Part model, mm, in its own coordinate system. A direction names the side the tool comes from. Round coordinates to 2 decimals unless told otherwise and drop trailing zeros. Write each loop counter-clockwise with the first axis right and the second up, starting at its lowest first coordinate (ties: lowest second). Pieces come first, ordered by that corner, then holes. Notation, with made-up numbers: M -11.75,-22.5 L 47.25,-22.5 A27 ccw 47.25,0.5 Z; hole C 0.25,54 d5. An arc over 180 degrees is marked long. One line per question, with ' | ' between items. Start each with the question number.
1) Wall check: probe 1 along Z at (x, y) = (68, 7); probe 2 along X at (y, z) = (18, -121.5); probe 3 along Z at (x, y) = (68.35, 7.5). Give the ranges that are in metal, low to high. Write a range as [from, to].
2) Drop flat-ended pins along their axis: pin 1 Ø1.5 at (x, z) = (77.5, -23) entering from +Y; pin 2 Ø1 at (x, y) = (96.5, 8.5) entering from -Z; pin 3 Ø4.5 at (x, y) = (45.5, 8) entering from -Z; pin 4 Ø3 at (y, z) = (7.5, -31.25) entering from -X. Give the stop position or say it passes through.
3) Mould opens along Z. For faces 1 (the face through (113, 10, -98.995)), 2 (the face through (69, 7, -138)), 3 (the face through (58, 2, -170)), 4 (the face through (75.29, 7, -100)) say: pulls with the +Z half, pulls with the -Z half, needs draft (parallel to the pull), parting line crosses it, or undercut.
4) Saw through at C-C (z = -122.5). List the corners of the cut face in (x, y).
5) Saw through at B-B (y = 26.5). List the corners of the cut face in (x, z), plus the area to 3 significant figures.
6) Tool access for faces 5 (the face through (45, 7, -48)), 6 (the face through (69.5, 6, -156)), 7 (the face through (112.782, 26.678, -66.163)), 8 (the face through (43.5, 7, -151)), 9 (the face through (96, 7, -102.576)): list every direction of +Z, -Z, +X, -X, +Y, -Y with a clear straight run to the whole face (end or side of a thin tool).
```python
from build123d import *

# Parameters (mm, degrees)
SKETCH1_W                  = 110.5
SKETCH1_H                  = 170
SKETCH1_W_2                = 4.5
BOSS_EXTRUDE1_DEPTH        = 4
SKETCH1_4_W                = 4.5
SKETCH1_4_H                = 170
BOSS_EXTRUDE2_DEPTH        = 50
CUT_EXTRUDE1_DEPTH         = 4.5
SALIENTE_EXTRUIR1_DEPTH    = 7
SALIENTE_EXTRUIR2_DEPTH    = 7
CORTAR_EXTRUIR1_DEPTH      = 31
CORTAR_EXTRUIR1_DEPTH_BACK = 7
CORTAR_EXTRUIR2_DEPTH      = 2
CHAFL_N1_SIZE              = 4
CHAFL_N2_SIZE              = 4
CROQUIS5_R                 = 2.5
CORTAR_EXTRUIR3_DEPTH      = 23.7
CHAFL_N3_SIZE              = 4
SALIENTE_EXTRUIR4_DEPTH    = 7
CROQUIS8_W                 = 12
CROQUIS8_H                 = 8
CORTAR_EXTRUIR4_DEPTH      = 7
REDONDEO1_R                = 2


with BuildPart() as part:
    # Sketch1 → Boss-Extrude1 (new body)
    with BuildSketch(Plane(origin=(0, 0, 0), x_dir=(1, 0, 0), z_dir=(0, 1, 0))):
        with Locations((59.75, 85)):
            Rectangle(SKETCH1_W, SKETCH1_H)
        with Locations((2.25, 85)):
            Rectangle(SKETCH1_W_2, SKETCH1_H)
    extrude(amount=BOSS_EXTRUDE1_DEPTH)

    # Sketch1<4> → Boss-Extrude2 (add)
    with BuildSketch(Plane(origin=(0, 0, 0), x_dir=(1, 0, 0), z_dir=(0, 1, 0))):
        with Locations((2.25, 85)):
            Rectangle(SKETCH1_4_W, SKETCH1_4_H)
    boss_extrude2 = extrude(amount=BOSS_EXTRUDE2_DEPTH)

    # Sketch2 → Cut-Extrude1 (cut)
    with BuildSketch(Plane.ZY):
        Polygon((-134.204014838, 50), (-170, 4), (-182.392562203, 4), (-182.392562203, 57.402643918), (5.745866014, 57.402643918), (5.745866014, 4), (0, 4), align=None)
    cut_extrude1 = extrude(amount=-CUT_EXTRUDE1_DEPTH, mode=Mode.SUBTRACT)

    # Mirror1: Boss-Extrude2, Cut-Extrude1 across plane
    add(boss_extrude2.mirror(Plane(origin=(57.5, 0, 0), x_dir=(0, 0, 1), z_dir=(1, 0, 0))))
    add(cut_extrude1.mirror(Plane(origin=(57.5, 0, 0), x_dir=(0, 0, 1), z_dir=(1, 0, 0))), mode=Mode.SUBTRACT)

    # Sketch3 → Saliente-Extruir1 (add)
    with BuildSketch(Plane(origin=(0, 4, 0), x_dir=(1, 0, 0), z_dir=(0, 1, 0))):
        Polygon((57.5, 160), (47.5, 160), (47.5, 142), (47.5, 138), (43.5, 138), (43.5, 164), (57.5, 164), align=None)
    saliente_extruir1 = extrude(amount=SALIENTE_EXTRUIR1_DEPTH)

    # Croquis1 → Saliente-Extruir2 (add)
    with BuildSketch(Plane(origin=(0, 4, 0), x_dir=(1, 0, 0), z_dir=(0, 1, 0))):
        Polygon((57.5, 26), (57.5, 22), (43.5, 22), (43.5, 48), (47.5, 48), (47.5, 26), align=None)
    saliente_extruir2 = extrude(amount=SALIENTE_EXTRUIR2_DEPTH)

    # Simetría1: Saliente-Extruir1, Saliente-Extruir2 across plane
    add(saliente_extruir1.mirror(Plane(origin=(57.5, 11, -164), x_dir=(0, 0, 1), z_dir=(-1, 0, 0))))
    add(saliente_extruir2.mirror(Plane(origin=(57.5, 11, -164), x_dir=(0, 0, 1), z_dir=(-1, 0, 0))))

    # Croquis2 → Cortar-Extruir1 (cut, two sides: drawn at the far end of the back side and taken through both)
    with BuildSketch(Plane(origin=(47.5, 0, 0), x_dir=(0, 0, -1), z_dir=(1, 0, 0)).offset(-CORTAR_EXTRUIR1_DEPTH_BACK)):
        with BuildLine():
            Line((31.25, 9.974873734), (32.487436867, 8.737436867))
            ThreePointArc((32.487436867, 8.737436867), (31.25, 5.75), (30.012563133, 8.737436867))
            Line((30.012563133, 8.737436867), (31.25, 9.974873734))
        make_face()
        with BuildLine():
            Line((154.75, 9.974873734), (155.987436867, 8.737436867))
            ThreePointArc((155.987436867, 8.737436867), (154.75, 5.75), (153.512563133, 8.737436867))
            Line((153.512563133, 8.737436867), (154.75, 9.974873734))
        make_face()
    extrude(amount=CORTAR_EXTRUIR1_DEPTH + CORTAR_EXTRUIR1_DEPTH_BACK, mode=Mode.SUBTRACT)

    # Croquis4 → Cortar-Extruir2 (cut)
    with BuildSketch(Plane(origin=(71.5, 0, 0), x_dir=(0, 0, -1), z_dir=(1, 0, 0))):
        Polygon((158.069764048, 7.5), (156.409882024, 10.375), (153.090117976, 10.375), (151.430235952, 7.5), (153.090117976, 4.625), (156.409882024, 4.625), align=None)
        Polygon((29.590117976, 4.625), (27.930235952, 7.5), (29.590117976, 10.375), (32.909882024, 10.375), (34.569764048, 7.5), (32.909882024, 4.625), align=None)
    extrude(amount=-CORTAR_EXTRUIR2_DEPTH, mode=Mode.SUBTRACT)

    # Chaflán1
    chafl_n1_edges = [part.edges().sort_by_distance(p)[0] for p in [
        (57.5, 11, -26),
    ]]
    chamfer(chafl_n1_edges, length=CHAFL_N1_SIZE - 0.0001)  # a hair under: the kernel refuses the full size

    # Chaflán2
    chafl_n2_edges = [part.edges().sort_by_distance(p)[0] for p in [
        (57.5, 11, -160),
    ]]
    chamfer(chafl_n2_edges, length=CHAFL_N2_SIZE - 0.0001)  # a hair under: the kernel refuses the full size

    # Croquis5 → Cortar-Extruir3 (cut)
    with BuildSketch(Plane(origin=(0, 4, 0), x_dir=(1, 0, 0), z_dir=(0, 1, 0))):
        with Locations(Location((33.545716199, 107.830838948, 0), (0, 0, 270))):
            Circle(CROQUIS5_R)
        with Locations(Location((57.5, 51.866184435, 0), (0, 0, 270))):
            Circle(CROQUIS5_R)
        with Locations(Location((81.454283801, 107.830838948, 0), (0, 0, 270))):
            Circle(CROQUIS5_R)
    extrude(amount=-CORTAR_EXTRUIR3_DEPTH, mode=Mode.SUBTRACT)

    # Chaflán3
    chafl_n3_edges = [part.edges().sort_by_distance(p)[0] for p in [
        (57.5, 0, 0),
    ]]
    chamfer(chafl_n3_edges, length=CHAFL_N3_SIZE - 0.0001)  # a hair under: the kernel refuses the full size

    # Saliente-Extruir3: read off the stored shape, not the designer's step
    # Saliente-Extruir3: loft between two sections, ruled curve by curve
    saliente_extruir3_from = [
        Edge.make_line((89.622165017, 4, -44.992823986), (87.622165017, 4, -44.990685532)),
        Edge.make_line((89.66503142, 4, -53.010916957), (89.622165017, 4, -44.992823986)),
        Edge.make_line((89.66503142, 4, -53.010916957), (97.363741989, 4, -53.010916957)),
        Edge.make_line((97.363741989, 4, -53.010916957), (97.363741989, 4, -44.990685532)),
        Edge.make_line((97.363741989, 4, -44.990685532), (99.363741989, 4, -44.990685532)),
        Edge.make_line((99.363741989, 4, -44.990685532), (99.363741989, 4, -55.010916957)),
        Edge.make_line((99.363741989, 4, -55.010916957), (87.622165017, 4, -55.010916957)),
        Edge.make_line((87.622165017, 4, -44.990685532), (87.622165017, 4, -55.010916957)),
    ]
    saliente_extruir3_to = [
        Edge.make_line((89.622165017, 8.969440836, -41.812469009), (87.622165017, 8.969440836, -41.810330556)),
        Edge.make_line((89.66503142, 8.969440836, -49.83056198), (89.622165017, 8.969440836, -41.812469009)),
        Edge.make_line((89.66503142, 8.969440836, -49.83056198), (97.363741989, 8.969440836, -49.83056198)),
        Edge.make_line((97.363741989, 8.969440836, -49.83056198), (97.363741989, 8.969440836, -41.810330556)),
        Edge.make_line((97.363741989, 8.969440836, -41.810330556), (99.363741989, 8.969440836, -41.810330556)),
        Edge.make_line((99.363741989, 8.969440836, -41.810330556), (99.363741989, 8.969440836, -51.83056198)),
        Edge.make_line((99.363741989, 8.969440836, -51.83056198), (87.622165017, 8.969440836, -51.83056198)),
        Edge.make_line((87.622165017, 8.969440836, -41.810330556), (87.622165017, 8.969440836, -51.83056198)),
    ]
    saliente_extruir3 = Solid(Shell([*[Face.make_surface_from_curves(saliente_extruir3_from[k], saliente_extruir3_to[k]) for k in range(8)], Face(Wire(saliente_extruir3_from)), Face(Wire(saliente_extruir3_to))]))
    add(saliente_extruir3)

    # Croquis7 → Saliente-Extruir4 (add)
    with BuildSketch(Plane(origin=(0, 4, 0), x_dir=(1, 0, 0), z_dir=(0, 1, 0))):
        with BuildLine():
            Line((93.557674933, 100.575775557), (95.79024416, 100.575775557))
            Line((95.79024416, 100.575775557), (97.79024416, 100.575775557))
            Line((97.79024416, 100.575775557), (97.79024416, 102.575775557))
            Line((97.79024416, 102.575775557), (94.59024416, 102.575775557))
            ThreePointArc((94.59024416, 102.575775557), (92.49024416, 103.475775557), (90.39024416, 102.575775557))
            Line((90.39024416, 102.575775557), (75.29024416, 102.575775557))
            Line((75.29024416, 102.575775557), (75.29024416, 97.575775557))
            Line((75.29024416, 97.575775557), (77.29024416, 97.575775557))
            Line((77.29024416, 97.575775557), (77.29024416, 100.575775557))
            Line((77.29024416, 100.575775557), (80.20924649, 100.575775557))
            Line((80.20924649, 100.575775557), (91.59024416, 100.575775557))
            ThreePointArc((91.59024416, 100.575775557), (92.49024416, 99.675775557), (93.39024416, 100.575775557))
            Line((93.39024416, 100.575775557), (93.557674933, 100.575775557))
        make_face()
        with BuildLine():
            Line((94.726312137, 74.375775557), (97.79024416, 74.375775557))
            Line((97.79024416, 74.375775557), (97.79024416, 76.375775557))
            Line((97.79024416, 76.375775557), (95.79024416, 76.375775557))
            Line((95.79024416, 76.375775557), (93.39024416, 76.375775557))
            ThreePointArc((93.39024416, 76.375775557), (92.49024416, 77.275775557), (91.59024416, 76.375775557))
            Line((91.59024416, 76.375775557), (83.611986998, 76.375775557))
            Line((83.611986998, 76.375775557), (77.29024416, 76.375775557))
            Line((77.29024416, 76.375775557), (77.29024416, 79.375775557))
            Line((77.29024416, 79.375775557), (75.29024416, 79.375775557))
            Line((75.29024416, 79.375775557), (75.29024416, 74.375775557))
            Line((75.29024416, 74.375775557), (90.254176182, 74.375775557))
            ThreePointArc((90.254176182, 74.375775557), (92.49024416, 73.375775557), (94.726312137, 74.375775557))
        make_face()
    extrude(amount=SALIENTE_EXTRUIR4_DEPTH)

    # Croquis8 → Cortar-Extruir4 (cut)
    with BuildSketch(Plane.ZY.offset(-110.5)):
        with Locations((-92.994977689, 10.20633678)):
            Rectangle(CROQUIS8_W, CROQUIS8_H)
    extrude(amount=-CORTAR_EXTRUIR4_DEPTH, mode=Mode.SUBTRACT)

    # Redondeo1
    redondeo1_edges = [part.edges().sort_by_distance(p)[0] for p in [
        (112.75, 14.20633678, -98.994977689),
        (112.75, 14.20633678, -86.994977689),
        (112.75, 6.20633678, -86.994977689),
        (112.75, 6.20633678, -98.994977689),
    ]]
    fillet(redondeo1_edges, radius=REDONDEO1_R)


solid = part.part
```
Answer key:
1) probe 1: z = [-164, -156.43], [-153.07, -138], [-48, -32.93], [-29.57, -22] | probe 2: x = [0, 4.5], [110.5, 115] | probe 3: z = [-164, -156.5], [-153, -138], [-48, -33], [-29.5, -22]
2) pin 1: stops at y = 4 | pin 2: stops at z = -102.58 | pin 3: stops at z = -164 | pin 4: stops at x = 0
3) face 1: undercut | face 2: undercut | face 3: pulls with the -Z half | face 4: needs draft
4) outline: M 0,0 L 115,0 L 115,45.99 L 110.5,45.99 L 110.5,4 L 4.5,4 L 4.5,45.99 L 0,45.99 Z
5) outline: M 0,-152.49 L 4.5,-152.49 L 4.5,-65.64 L 0,-65.64 Z; M 110.5,-152.49 L 115,-152.49 L 115,-65.64 L 110.5,-65.64 Z | area: 782 mm2
6) face 5: +Y | face 6: none | face 7: +Z, +X, -X, +Y | face 8: +Z, -Z, +Y | face 9: -Z, +Y
